Geometry: see drawing. Coordinates: mm, zero at the bounding-box minimum. A direction names the side the tool comes from. Coordinates: 2 decimals unless noted, no trailing zeros. Loops run counter-clockwise (first coordinate to the right, second up) from the corner with the lowest first, then second, coordinate; pieces in that order, holes last.
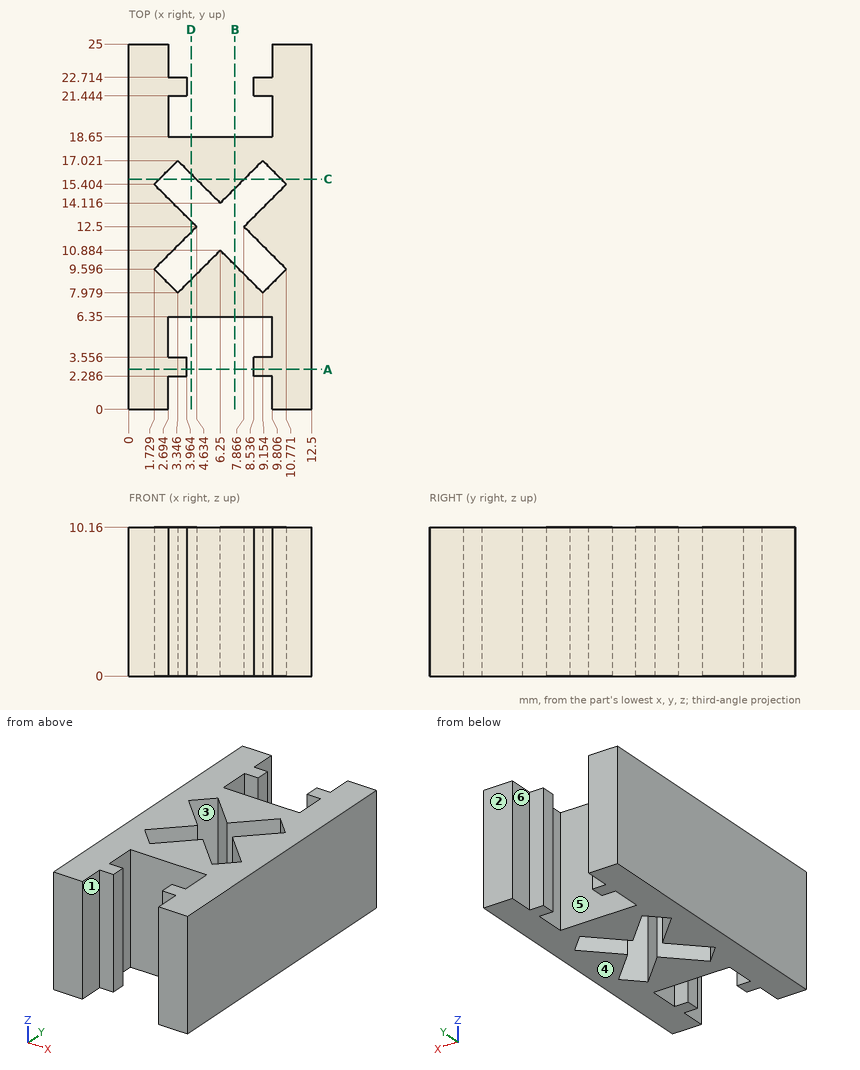
Item 1: Section query C-C (y = 15.75). Output: boundary loops of the cut face in (x, z) (1 decimal).
Result:
outline: (0, 0) - (2.1, 0) - (2.1, 10.2) - (0, 10.2) - close; (4.6, 0) - (7.9, 0) - (7.9, 10.2) - (4.6, 10.2) - close; (10.4, 0) - (12.5, 0) - (12.5, 10.2) - (10.4, 10.2) - close
Item 2: Section query B-B (x = 7.25). Output: boundary loops of the cut face in (y, z).
Result:
outline: (6.35, 0) - (9.88, 0) - (9.88, 10.16) - (6.35, 10.16) - close; (15.12, 0) - (18.65, 0) - (18.65, 10.16) - (15.12, 10.16) - close
Item 3: Reachability of the marked faces 4, 5 and 6 from +Z, -Z, +X, -X, +Y, -Y: full face, straight path, thin tool, end or side. Return the list, or none.
Result:
face 4: -Z, +X, -X, +Y, -Y
face 5: +Z, -Z
face 6: +Z, -Z, +Y
Item 4: Line query: L1, parallel to X at y = 20.5, z = 8.75; L2, parallel to X at y = 22, z = 5.5; L3, parallel to X at y = 16.75, z = 6 (1 decimal). Output: solid intervals per line, ascending.
Result:
L1: x = 0 to 2.69, 9.81 to 12.5
L2: x = 0 to 3.96, 8.54 to 12.5
L3: x = 0 to 3.1, 3.6 to 8.9, 9.4 to 12.5
Item 5: Mould query, pull axis Y, two halves, no side actions, for the marked faces 1, 2 and 3. Classes: +Y half, -Y half, draft (parallel to the pull), parting line (faces both ways), or undercut.
Result:
face 1: draft
face 2: +Y half
face 3: undercut
Item 6: Section query A-A (y = 2.75). Output: boundary loops of the cut face in (x, z).
Result:
outline: (0, 0) - (3.96, 0) - (3.96, 10.16) - (0, 10.16) - close; (8.54, 0) - (12.5, 0) - (12.5, 10.16) - (8.54, 10.16) - close
Item 7: Contact query for flat-ended pins moving along their axis: P1, Ø1, axis at x = 6, z = 2.5, coming from the -Y side; P2, Ø1, axis at x = 3.5, z = 3.5, coming from the -Y side. Output: stop coordinate, or through.
Result:
P1: stops at y = 6.35
P2: stops at y = 2.29
Item 8: Section query D-D (x = 4.25). Output: boundary loops of the cut face in (y, z).
Result:
outline: (6.35, 0) - (8.88, 0) - (8.88, 10.16) - (6.35, 10.16) - close; (12.12, 0) - (12.88, 0) - (12.88, 10.16) - (12.12, 10.16) - close; (16.12, 0) - (18.65, 0) - (18.65, 10.16) - (16.12, 10.16) - close
